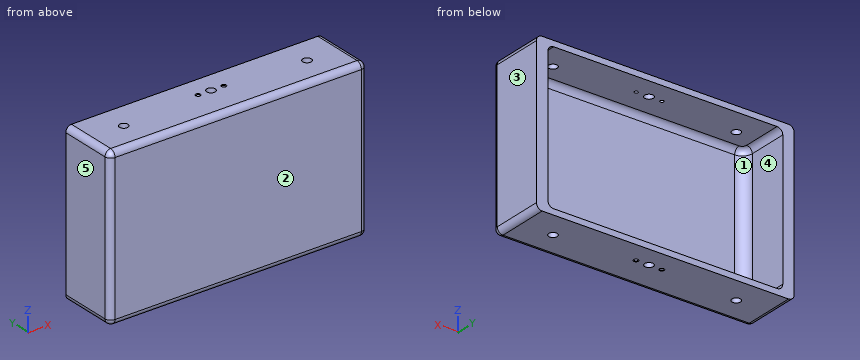
```python
from build123d import *

# Parameters (mm, degrees)
ESQUISSE1_W                   = 90
ESQUISSE1_H                   = 20
ESQUISSE1_R                   = 1.5
BOSS_EXTRU_1_DEPTH            = 2
ESQUISSE2_W                   = 90
ESQUISSE2_H                   = 20
BOSS_EXTRU_2_DEPTH            = 51
ENL_V_MAT_EXTRU_2_DEPTH       = 51
ESQUISSE6_W                   = 90
ESQUISSE6_H                   = 20
ESQUISSE6_R                   = 1.5
BOSS_EXTRU_4_DEPTH            = 2
TROU_TARAUD_M1_61_D           = 1.25
TROU_TARAUD_M1_61_DEPTH       = 2
TROU_TARAUD_M1_61_CSINK_D     = 1.65
TROU_TARAUD_M1_61_CSINK_ANGLE = 90
TROU_TARAUD_M1_62_D           = 1.25
TROU_TARAUD_M1_62_DEPTH       = 2
TROU_TARAUD_M1_62_CSINK_D     = 1.65
TROU_TARAUD_M1_62_CSINK_ANGLE = 90
CONG_1_R                      = 2
CONG_2_R                      = 2
CONG_3_R                      = 2
CONG_4_R                      = 2


with BuildPart() as part:
    # Esquisse1 → Boss.-Extru.1 (new body)
    with BuildSketch(Plane.XY):
        with Locations((0, 10)):
            Rectangle(ESQUISSE1_W, ESQUISSE1_H)
        with Locations((-32, 10.5)):
            Circle(ESQUISSE1_R, mode=Mode.SUBTRACT)
        with Locations((32, 10.5)):
            Circle(ESQUISSE1_R, mode=Mode.SUBTRACT)
        with Locations((0, 12.5)):
            Circle(ESQUISSE1_R, mode=Mode.SUBTRACT)
    extrude(amount=BOSS_EXTRU_1_DEPTH)

    # Esquisse2 → Boss.-Extru.2 (add)
    with BuildSketch(Plane.XY.offset(2)):
        with Locations((0, 10)):
            Rectangle(ESQUISSE2_W, ESQUISSE2_H)
    extrude(amount=BOSS_EXTRU_2_DEPTH)

    # Esquisse4 → Enlèv. mat.-Extru.2 (cut)
    with BuildSketch(Plane.XY.offset(53)):
        with BuildLine():
            Line((-37.5, 2.5), (37.5, 2.5))
            ThreePointArc((37.5, 2.5), (39.974873734, 3.525126266), (41, 6))
            Line((41, 6), (41, 20))
            Line((41, 20), (-41, 20))
            Line((-41, 20), (-41, 6))
            ThreePointArc((-41, 6), (-39.974873734, 3.525126266), (-37.5, 2.5))
        make_face()
    extrude(amount=-ENL_V_MAT_EXTRU_2_DEPTH, mode=Mode.SUBTRACT)

    # Esquisse6 → Boss.-Extru.4 (add)
    with BuildSketch(Plane.XY.offset(53)):
        with Locations((0, 10)):
            Rectangle(ESQUISSE6_W, ESQUISSE6_H)
        with Locations((32, 10.5)):
            Circle(ESQUISSE6_R, mode=Mode.SUBTRACT)
        with Locations((0, 12.5)):
            Circle(ESQUISSE6_R, mode=Mode.SUBTRACT)
        with Locations((-32, 10.5)):
            Circle(ESQUISSE6_R, mode=Mode.SUBTRACT)
    extrude(amount=BOSS_EXTRU_4_DEPTH)

    # Trou taraudé M1.61
    with Locations(Plane.XY.offset(55)):
        with Locations((-4.5, 12.5), (4.5, 12.5)):
            CounterSinkHole(TROU_TARAUD_M1_61_D / 2, TROU_TARAUD_M1_61_CSINK_D / 2, depth=TROU_TARAUD_M1_61_DEPTH, counter_sink_angle=TROU_TARAUD_M1_61_CSINK_ANGLE)

    # Trou taraudé M1.62
    with Locations(Plane(origin=(0, 0, 0), x_dir=(-1, 0, 0), z_dir=(0, 0, -1))):
        with Locations((-4.5, 12.497038502), (4.5, 12.497038502)):
            CounterSinkHole(TROU_TARAUD_M1_62_D / 2, TROU_TARAUD_M1_62_CSINK_D / 2, depth=TROU_TARAUD_M1_62_DEPTH, counter_sink_angle=TROU_TARAUD_M1_62_CSINK_ANGLE)

    # Congé1
    cong_1_edges = [part.edges().sort_by_distance(p)[0] for p in [
        (-39.974873734, 3.525126266, 2),
        (-41, 13, 2),
        (41, 13, 2),
        (39.974873734, 3.525126266, 2),
        (0, 2.5, 2),
    ]]
    fillet(cong_1_edges, radius=CONG_1_R)

    # Congé2
    cong_2_edges = [part.edges().sort_by_distance(p)[0] for p in [
        (-39.974873734, 3.525126266, 53),
        (0, 2.5, 53),
        (39.974873734, 3.525126266, 53),
        (41, 13, 53),
        (-41, 13, 53),
    ]]
    fillet(cong_2_edges, radius=CONG_2_R)

    # Congé3
    cong_3_edges = [part.edges().sort_by_distance(p)[0] for p in [
        (0, 0, 0),
        (0, 0, 55),
        (45, 0, 27.5),
        (-45, 0, 27.5),
    ]]
    fillet(cong_3_edges, radius=CONG_3_R)

    # Congé4
    # the kernel refuses this fillet: 2 mm, written as the material it takes off along each edge
    with BuildSketch(Plane(origin=(43, 2, 53), x_dir=(0, 0, 1), z_dir=(1, 0, 0))) as cong_4_piece_1_section:
        Polygon((0, 0), (CONG_4_R, 0), (CONG_4_R, CONG_4_R), (0, CONG_4_R), align=None)
    cong_4_piece_1 = extrude(amount=CONG_4_R, mode=Mode.PRIVATE)
    cong_4_piece_1 = cong_4_piece_1 - Plane(origin=(43, 2, 53), x_dir=(0, 0.7071067811865475, -0.7071067811865475), z_dir=(1, 0, 0)) * Sphere(CONG_4_R, mode=Mode.PRIVATE)
    add(cong_4_piece_1, mode=Mode.SUBTRACT)
    with BuildSketch(Plane(origin=(43, 2, 2), x_dir=(1, 0, 0), z_dir=(0, 0, -1))) as cong_4_piece_2_section:
        Polygon((0, 0), (CONG_4_R, 0), (CONG_4_R, CONG_4_R), (0, CONG_4_R), align=None)
    cong_4_piece_2 = extrude(amount=CONG_4_R, mode=Mode.PRIVATE)
    cong_4_piece_2 = cong_4_piece_2 - Plane(origin=(43, 2, 2), x_dir=(-0.7071067811865474, 0.7071067811865477, 0), z_dir=(0, 0, -1)) * Sphere(CONG_4_R, mode=Mode.PRIVATE)
    add(cong_4_piece_2, mode=Mode.SUBTRACT)
    with BuildSketch(Plane(origin=(-43, 2, 53), x_dir=(0, 0, 1), z_dir=(-1, 0, 0))) as cong_4_piece_3_section:
        Polygon((0, 0), (CONG_4_R, 0), (CONG_4_R, -CONG_4_R), (0, -CONG_4_R), align=None)
    cong_4_piece_3 = extrude(amount=CONG_4_R, mode=Mode.PRIVATE)
    cong_4_piece_3 = cong_4_piece_3 - Plane(origin=(-43, 2, 53), x_dir=(0, 0.7071067811865475, -0.7071067811865475), z_dir=(-1, 0, 0)) * Sphere(CONG_4_R, mode=Mode.PRIVATE)
    add(cong_4_piece_3, mode=Mode.SUBTRACT)
    with BuildSketch(Plane(origin=(-43, 2, 2), x_dir=(-1, 0, 0), z_dir=(0, 0, -1))) as cong_4_piece_4_section:
        Polygon((0, 0), (CONG_4_R, 0), (CONG_4_R, -CONG_4_R), (0, -CONG_4_R), align=None)
    cong_4_piece_4 = extrude(amount=CONG_4_R, mode=Mode.PRIVATE)
    cong_4_piece_4 = cong_4_piece_4 - Plane(origin=(-43, 2, 2), x_dir=(0.7071067811865474, 0.7071067811865477, 0), z_dir=(0, 0, -1)) * Sphere(CONG_4_R, mode=Mode.PRIVATE)
    add(cong_4_piece_4, mode=Mode.SUBTRACT)
    with BuildSketch(Plane(origin=(45, 2, 55), x_dir=(0, 0, -1), z_dir=(0, 1, 0)), Plane(origin=(-45, 25, 55), x_dir=(0, 0, -1), z_dir=(0, -1, 0))) as cong_4_piece_5:
        with BuildLine():
            CenterArc((CONG_4_R, CONG_4_R), CONG_4_R, 180, 90)
            Line((0, CONG_4_R), (0, 0))
            Line((0, 0), (CONG_4_R, 0))
        make_face()
    extrude(amount=23, mode=Mode.SUBTRACT)
    with BuildSketch(Plane(origin=(45, 25, 0), x_dir=(-1, 0, 0), z_dir=(0, -1, 0)), Plane(origin=(-45, 2, 0), x_dir=(1, 0, 0), z_dir=(0, 1, 0))) as cong_4_piece_6:
        with BuildLine():
            CenterArc((CONG_4_R, -CONG_4_R), CONG_4_R, 90, 90)
            Line((0, -CONG_4_R), (0, 0))
            Line((0, 0), (CONG_4_R, 0))
        make_face()
    extrude(amount=23, mode=Mode.SUBTRACT)


solid = part.part
```
Source: CAD feature listing. Evaluate the final solid. Frame: model axes, mm. Face numbers are marked on the shaded views. A direction names the side the tool comes from. Coordinates: 2 decimals unless noted, no trailing zeros. Loops run counter-clockwise (first coordinate to the right, second up) from the corner with the lowest first, then second, coordinate; pieces in that order, holes last. Notation, with made-up numbers: M 18.5,-29.5 L 44.5,-29.5 A10 ccw 44.5,-13.5 Z; hole C 46.25,-4.5 d4. An arc over 180 degrees is marked long. Use a Markdown table: item, result. Add a question column.
Q1. Section query C-C, the plane z = 39. Return loops of the section in (x, y).
Q2. Section query B-B, the plane x = 20.5. Return loops of the section in (y, z), and give its area (4 significant figures).
Q3. Section query A-A, the plane x = 32. Return loops of the section in (y, z).
Q4. First-contact query: pin 1 (1.6 mm diameter, centred on x = 4.5, y = 12.5, fed in from +Z) (3 decimals); pin 2 (1.4 mm diameter, centred on x = -4.5, y = 12.5, fed in from -Z); pin 3 (23.5 mm diameter, centred on x = -13, z = 36, fed in from +Y). Flat tips, straight axial feed; report the tip coordinate or a pass-through.
Q5. Access query for the marked faces 1 and 2. Directions: +Z, -Z, +X, -X, +Y, -Y. A direction counts if a zero-diameter tool reaches every point of the face in a straight line with its end or side. Return the directions, or none.
Q6. Material intervals for L1, parallel to Z at x = 20.5, y = 10; L2, parallel to X at y = 16, z = 49; L3, parallel to Y at x = 32, z = 48, sorted ascending.
Q7. Draft query along X for the marked faces 3, 4 and 5. Return one class per face: pulls with the +X half, pulls with the -X half, needs draft (parallel to the pull), parting line crosses it, or undercut.
Result:
| question | item | result |
|---|---|---|
| 1 | outline | M -45,2 A2 ccw -43,0 L 43,0 A2 ccw 45,2 L 45,20 L 41,20 L 41,6 A3.5 cw 37.5,2.5 L -37.5,2.5 A3.5 cw -41,6 L -41,20 L -45,20 Z |
| 2 | outline | M 0,2 A2 ccw 2,0 L 20,0 L 20,2 L 4.5,2 A2 cw 2.5,4 L 2.5,51 A2 cw 4.5,53 L 20,53 L 20,55 L 2,55 A2 ccw 0,53 Z |
| 2 | area | 207.5 mm2 |
| 3 | outline | M 0,2 A2 ccw 2,0 L 9,0 L 9,2 L 4.5,2 A2 cw 2.5,4 L 2.5,51 A2 cw 4.5,53 L 9,53 L 9,55 L 2,55 A2 ccw 0,53 Z; M 12,0 L 20,0 L 20,2 L 12,2 Z; M 12,53 L 20,53 L 20,55 L 12,55 Z |
| 4 | pin 1 | stops at z = 54.975 |
| 4 | pin 2 | stops at z = 0.12 |
| 4 | pin 3 | stops at y = 2.5 |
| 5 | face 1 | +Y |
| 5 | face 2 | +Z, -Z, +X, -X, -Y |
| 6 | L1 | z = 0 to 2, 53 to 55 |
| 6 | L2 | x = -45 to -41, 41 to 45 |
| 6 | L3 | y = 0 to 2.5 |
| 7 | face 3 | pulls with the +X half |
| 7 | face 4 | undercut |
| 7 | face 5 | pulls with the -X half |
